Autodesk Inventor part; units mm, degrees
ref_plane "YZ Plane" through (0, 0, 0) normal (1, 0, 0) x (0, 1, 0)
ref_plane "XZ Plane" through (0, 0, 0) normal (0, 1, 0) x (-1, 0, 0)
ref_plane "XY Plane" through (0, 0, 0) normal (0, 0, 1) x (1, 0, 0)
sketch "Sketch4" plane through (0, 0, 0) normal (0, 0, 1) x (1, 0, 0)
  line L0 (0, 0) -> (-8, 0)
  line L1 (-8, 0) -> (-8, 8)
  line L2 (-8, 8) -> (0, 8)
  line L3 (0, 8) -> (0, 0)
  dimension "d30" = 8
  dimension "d31" = 8
extrude "Extrusion6" add sketch "Sketch4" along normal blind 10
sketch "Sketch6" plane through (0, 0, 10) normal (0, 0, 1) x (1, 0, 0)
  line L0 (-4, 4) -> (-6.8, 4)
  line L1 (-6.8, 4) -> (-6.8, 6.8)
  line L2 (-6.8, 6.8) -> (-4, 6.8)
  line L3 (-4, 6.8) -> (-4, 4)
  line L4 (-6.8, 6.8) -> (-1.2, 6.8)
  line L5 (-1.2, 6.8) -> (-1.2, 1.2)
  line L6 (-1.2, 1.2) -> (-6.8, 1.2)
  line L7 (-6.8, 1.2) -> (-6.8, 6.8)
  point P0 (0, 0)
  dimension "d40" = 2.8
  dimension "d41" = 2.8
  dimension "d42" = 5.6
  dimension "d43" = 5.6
extrude "Extrusion8" cut sketch "Sketch6" against normal blind 5
properties part number "Clip_MarkerHolderV1"
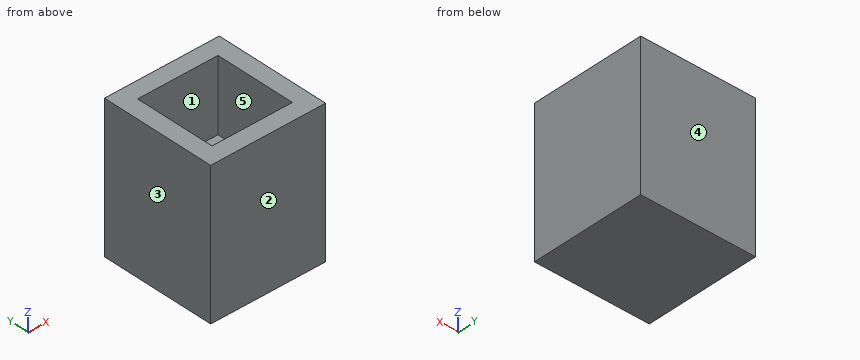
Here's how the part is built. I have some questions about the finished solid (model axes, mm). Face numbers are marked on the shaded views. A direction names the side the tool comes from. Give positions to 0.01 mm unless a question says otherwise; leave off trailing zeros. Loops run counter-clockwise (first coordinate to the right, second up) from the corner with the lowest first, then second, coordinate; pieces in that order, holes last. Notation, with made-up numbers: M 33.5,68 L 42.5,68 A24 cw 42.5,99 Z; hole C 56.5,-36.5 d1. An arc over 180 degrees is marked long. Put each result on its own line as item: value. Start each with the question number.
(1) I want a section at B-B on y = 2.25. Please give me the cut outline in (x, z).
(2) I want a section at A-A on z = 8.75. Please give me the cut outline in (x, y).
(3) I want a section at C-C on x = -5.5. Please give me the cut outline in (y, z).
(4) If we mould it in two halves opening along X, with no side actions, what happens to the marked faces 3, 4 and 5? For each: +X half, -X half, draft (parallel to the pull), parting line (faces both ways), or undercut.
(5) For the marked faces 1 and 2, which set-ups out of +Z, -Z, +X, -X, +Y, -Y let a thin tool reach every point of the face, with its end or its side?
(6) I need wall thicknesses on line 1 along X through (y, z) = (1.5, 7.75); line 2 along Y through (x, z) = (-6.75, 6.75); line 3 along Z through (x, y) = (-6.5, 3.25). Which ranges of each line are inside material? Lowest first, please. Write a range as [from, to].
(7) Will this pin go through, and if not, where does the flat tip stop? pin 1 Ø4 at (y, z) = (5, 8) entering from +X.
Answer block:
1. outline: M -8,0 L 0,0 L 0,10 L -1.2,10 L -1.2,5 L -6.8,5 L -6.8,10 L -8,10 Z
2. outline: M -8,0 L 0,0 L 0,8 L -8,8 Z; hole M -6.8,1.2 L -1.2,1.2 L -1.2,6.8 L -6.8,6.8 Z
3. outline: M 0,0 L 8,0 L 8,10 L 6.8,10 L 6.8,5 L 1.2,5 L 1.2,10 L 0,10 Z
4. face 3: -X half
4. face 4: draft
4. face 5: undercut
5. face 1: +Z
5. face 2: +Z, -Z, +X, -X, -Y
6. line 1: [-8, -6.8], [-1.2, 0]
6. line 2: [0, 1.2], [6.8, 8]
6. line 3: [0, 5]
7. pin 1: x = 0
